The drawing under review shows one solid part. Ordinate dimensions are in mm from its lowest x, y, z. A direction names the side the tool comes from. Round coordinates to 2 decimals unless told otherwise and drop trailing zeros. Order: outer loops, then holes, each group sorted by start corner. A loop starts at its lowest first (then second) coordinate and runs counter-clockwise, first axis right, second up. Notation, with made-up numbers: (72.5, -31) -> (123.5, -31) arc R12 cw to (123.5, -12) -> close; hole circle Ø2 at (-12.5, 72). An arc over 180 degrees is marked (long way). Put each result on its own line as item: value. Start each with the question number.
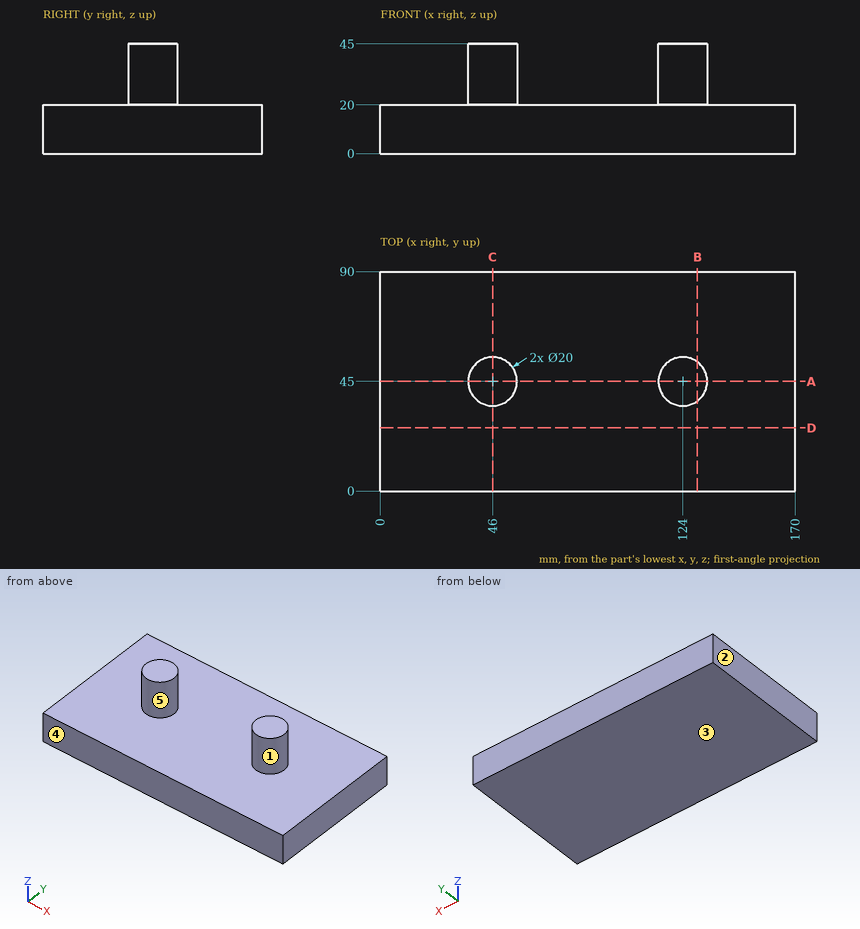
Item 1: Mouldability with a two-part tool opening along X and no side actions: class the marked faces 1, 2 and 3 as +X half, -X half, draft (parallel to the pull), parting line (faces both ways), or undercut.
Item 2: Insertion check: pin 1 Ø1 at (x, y) = (58, 33.5) entering from -Z; pin 2 Ø8 at (x, y) = (95, 40) entering from +Z; pin 3 Ø12 at (x, z) = (132, 31) entering from +Y. Each pin has a flat end and moves straight along its axis. Give the tip position at first contact, or say it passes through.
Item 3: Consider section B-B, the plane x = 130. Write out the cut boundary in (y, z), plus the area to 3 significant figures.
Item 4: Tool access review of the marked faces 4 and 5: name each direction out of +Z, -Z, +X, -X, +Y, -Y from which nothing blocks a thin tool from reaching the whole face with its end or side.
Item 5: Consider section A-A, the plane y = 45. Write out the cut boundary in (x, z), plus the area to 3 significant figures.
Item 6: For L1, parallel to Z at x = 35, y = 71; L2, parallel to X at y = 43.5, z = 29; L3, parallel to Y at x = 55, z = 28.5, list the stretches that pass through material, from the lowest coordinate up.
Item 7: Consider section C-C, the plane x = 46. Write out the cut boundary in (y, z).
Item 8: Consider section D-D, the plane y = 26. Write out the cut boundary in (x, z), plus the area to 3 significant figures.
Evaluation:
1. face 1: undercut
1. face 2: -X half
1. face 3: draft
2. pin 1: stops at z = 0
2. pin 2: stops at z = 20
2. pin 3: stops at y = 54.8
3. outline: (0, 0) -> (90, 0) -> (90, 20) -> (53, 20) -> (53, 45) -> (37, 45) -> (37, 20) -> (0, 20) -> close
3. area: 2,200 mm^2
4. face 4: +Z, -Z, +X, -X, -Y
4. face 5: +Z
5. outline: (0, 0) -> (170, 0) -> (170, 20) -> (134, 20) -> (134, 45) -> (114, 45) -> (114, 20) -> (56, 20) -> (56, 45) -> (36, 45) -> (36, 20) -> (0, 20) -> close
5. area: 4,400 mm^2
6. L1: z = 0 to 20
6. L2: x = 36.11 to 55.89, 114.11 to 133.89
6. L3: y = 40.64 to 49.36
7. outline: (0, 0) -> (90, 0) -> (90, 20) -> (55, 20) -> (55, 45) -> (35, 45) -> (35, 20) -> (0, 20) -> close
8. outline: (0, 0) -> (170, 0) -> (170, 20) -> (0, 20) -> close
8. area: 3,400 mm^2
